from build123d import *

# Parameters (mm, degrees)
BOSS_EXTRUDE1_DEPTH = 0.2
FILLET3_R           = 0.1
BOSS_EXTRUDE2_DEPTH = 1.3
FILLET4_R           = 0.1


with BuildPart() as part:
    # Sketch2 → Boss-Extrude1 (new body)
    with BuildSketch(Plane(origin=(0, 0, 0), x_dir=(1, 0, 0), z_dir=(0, 1, 0))):
        with BuildLine():
            Line((8.774632583, 14.872725815), (14.774632583, 14.872725815))
            ThreePointArc((14.774632583, 14.872725815), (17.274632583, 12.372725815), (14.774632583, 9.872725815))
            Line((14.774632583, 9.872725815), (8.774632583, 9.872725815))
            ThreePointArc((8.774632583, 9.872725815), (6.274632583, 12.372725815), (8.774632583, 14.872725815))
        make_face()
    extrude(amount=BOSS_EXTRUDE1_DEPTH)

    # Fillet3
    fillet3_edges = [part.edges().sort_by_distance(p)[0] for p in [
        (17.274632583, 0.2, -12.372725815),
        (11.774632583, 0.2, -14.872725815),
        (6.274632583, 0.2, -12.372725815),
        (11.774632583, 0.2, -9.872725815),
    ]]
    fillet(fillet3_edges, radius=FILLET3_R)

    # Sketch5 → Boss-Extrude2 (add)
    with BuildSketch(Plane(origin=(0, 0.2, 0), x_dir=(1, 0, 0), z_dir=(0, 1, 0))):
        with BuildLine():
            Line((8.774632583, 14.772725815), (14.774632583, 14.772725815))
            ThreePointArc((14.774632583, 14.772725815), (17.174632583, 12.372725815), (14.774632583, 9.972725815))
            Line((14.774632583, 9.972725815), (8.774632583, 9.972725815))
            ThreePointArc((8.774632583, 9.972725815), (6.374632583, 12.372725815), (8.774632583, 14.772725815))
        make_face()
    extrude(amount=BOSS_EXTRUDE2_DEPTH)

    # Fillet4
    fillet4_edges = [part.edges().sort_by_distance(p)[0] for p in [
        (6.374632583, 1.5, -12.372725815),
        (11.774632583, 1.5, -9.972725815),
        (17.174632583, 1.5, -12.372725815),
        (11.774632583, 1.5, -14.772725815),
    ]]
    fillet(fillet4_edges, radius=FILLET4_R)


solid = part.part
Verification items for the finished model (mm, model axes). A direction names the side the tool comes from. Give positions to 0.01 mm unless a question says otherwise; leave off trailing zeros. Write each loop counter-clockwise with the first axis right and the second up, starting at its lowest first coordinate (ties: lowest second). Pieces come first, ordered by that corner, then holes. Notation, with made-up numbers: M -31.75,58 L -16.75,58 A19 cw -16.75,76 Z; hole C 12,75.5 d6. An arc over 180 degrees is marked long. Put each result on its own line as item: value. Start each with the question number.
1. Set-up check for faces 1 (the face through (12, 0, -12)), 2 (the face through (17.174, 0.792, -12.426)): record each of +Z, -Z, +X, -X, +Y, -Y from which the full face is reachable in a straight line by a thin tool's end or side.
2. Scan lines: line 1 along Z through (x, y) = (11, 1.05); line 2 along X through (y, z) = (0.25, -12.45); line 3 along Z through (x, y) = (16.5, 0.85). Record each from-to range of solid material in increasing order. Write a range as [from, to].
3. Section check A-A (x = 13.25). Record the cut outline in (y, z).
4. Section check B-B (y = 0.6). Record the cut outline in (x, z).
5. Draft check along Z on faces 3 (the face through (12, 1, -14.773)), 4 (the face through (12, 1, -9.973)), 5 (the face through (12, 1.5, -12)), 6 (the face through (6.375, 0.792, -12.32)). Enter one of: +Z half, -Z half, draft (parallel to the pull), parting line (faces both ways), or undercut.
Answer list:
1. face 1: +Z, -Z, +X, -X, -Y
1. face 2: +X, +Y
2. line 1: [-14.77, -9.97]
2. line 2: [6.38, 17.17]
2. line 3: [-14.04, -10.7]
3. outline: M 0,-14.87 L 0.1,-14.87 A0.1 ccw 0.2,-14.77 L 1.4,-14.77 A0.1 ccw 1.5,-14.67 L 1.5,-10.07 A0.1 ccw 1.4,-9.97 L 0.2,-9.97 A0.1 ccw 0.1,-9.87 L 0,-9.87 Z
4. outline: M 8.77,-14.77 L 14.77,-14.77 A2.4 ccw 14.77,-9.97 L 8.77,-9.97 A2.4 ccw Z
5. face 3: -Z half
5. face 4: +Z half
5. face 5: draft
5. face 6: parting line
